Check sheet for the modelled part. Datum: model origin and axes. Units: mm. Face numbers are marked on the shaded views. A direction names the side the tool comes from. Round coordinates to 2 decimals unless told otherwise and drop trailing zeros. Write each loop counter-clockwise with the first axis right and the second up, starting at its lowest first coordinate (ties: lowest second). Pieces come first, ordered by that corner, then holes. Notation, with made-up numbers: (-36, 40) -> (8, 40) arc R26 ccw to (8, 66) -> close; hole circle Ø8 at (69.25, 27). An arc over 180 degrees is marked (long way). Write item = value, one per line.
from build123d import *

# Parameters (mm, degrees)
F2_DEPTH = 3.5
F4_DEPTH = 1
F6_DEPTH = 1.8
F8_DEPTH = 1.2
F9_R     = 3


with BuildPart() as f2:
    # F1 (on Top) → F2 (new body)
    with BuildSketch(Plane.XY):
        Polygon((48.5598316574, 13.5), (5.4801683426, 13.5), (27.0198316574, -13.5), align=None)
    extrude(amount=-F2_DEPTH)

    # F3 (on Top) → F4 (cut)
    with BuildSketch(Plane.XY):
        Polygon((44.7943471372, 11.7882982132), (6.8457046456, 11.7882982132), (25.8198775993, -11.9958558036), align=None)
    extrude(amount=-F4_DEPTH, mode=Mode.SUBTRACT)

    # F5 (on face) → F6 (join)
    with BuildSketch(Plane.XY):
        with BuildLine():
            ThreePointArc((2.8793278964, 3.7278809202), (3.7658696299, 2.8294612951), (4.3820146982, 1.7278809202))
            Line((4.3820146982, 1.7278809202), (14.8715565456, 1.7278809202))
            Line((14.8715565456, 1.7278809202), (17.594606702, -1.6854665007))
            Line((17.594606702, -1.6854665007), (4.3985029231, -1.6854665007))
            ThreePointArc((4.3985029231, -1.6854665007), (3.7999051439, -2.783585132), (2.9334215452, -3.6854665007))
            Line((2.9334215452, -3.6854665007), (19.1901373179, -3.6854665007))
            Line((19.1901373179, -3.6854665007), (25.8198775993, -11.9958558036))
            Line((25.8198775993, -11.9958558036), (44.7943471372, 11.7882982132))
            Line((44.7943471372, 11.7882982132), (6.8457046456, 11.7882982132))
            Line((6.8457046456, 11.7882982132), (13.2760259297, 3.7278809202))
            Line((13.2760259297, 3.7278809202), (2.8793278964, 3.7278809202))
        make_face()
        Polygon((5.4801683426, 13.5), (6.8457046456, 11.7882982132), (44.7943471372, 11.7882982132), (25.8198775993, -11.9958558036), (27.0198316574, -13.5), (48.5598316574, 13.5), align=None)
        with BuildLine():
            Line((-4.3820146982, 1.7278809202), (4.3820146982, 1.7278809202))
            ThreePointArc((4.3820146982, 1.7278809202), (3.7658696299, 2.8294612951), (2.8793278964, 3.7278809202))
            ThreePointArc((2.8793278964, 3.7278809202), (-1.2508065023, 4.5412672663), (-4.3820146982, 1.7278809202))
        make_face()
        with BuildLine():
            ThreePointArc((2.9334215452, -3.6854665007), (3.7999051439, -2.783585132), (4.3985029231, -1.6854665007))
            Line((4.3985029231, -1.6854665007), (-4.3985029231, -1.6854665007))
            ThreePointArc((-4.3985029231, -1.6854665007), (-1.2396031062, -4.5443381728), (2.9334215452, -3.6854665007))
        make_face()
    extrude(amount=F6_DEPTH)

    # F7 (on face) → F8 (join)
    with BuildSketch(Plane.XY.offset(1.8)):
        Polygon((48.5598316574, 13.5), (5.4801683426, 13.5), (13.2760259297, 3.7278809202), (14.8715565456, 1.7278809202), (17.594606702, -1.6854665007), (19.1901373179, -3.6854665007), (27.0198316574, -13.5), align=None)
    extrude(amount=F8_DEPTH)

    # F9
    f9_edges = [f2.edges().sort_by_distance(p)[0] for p in [
        (27.02, 13.5, 3),
        (27.02, 13.5, -3.5),
        (37.789832, 0, 3),
        (37.789832, 0, -3.5),
    ]]
    fillet(f9_edges, radius=F9_R)


solid = f2.part
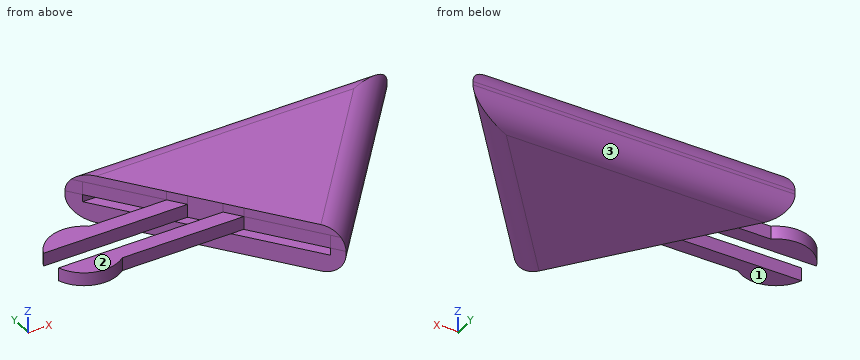
(1) Sectioned sample at B-B on x = 9.5. Enter the section's corners in (y, z), then the cut area to 3 significant figures.
Worked answers:
outline = (-3.69, 0) -> (-1.69, 0) -> (-1.69, 1.8) -> (-3.69, 1.8) -> close; (1.73, 0) -> (3.73, 0) -> (3.73, 1.8) -> (1.73, 1.8) -> close; (8.46, -3.5) -> (10.5, -3.5) arc R3 ccw to (13.5, -0.5) -> (13.5, 0) arc R3 ccw to (10.5, 3) -> (8.46, 3) -> (8.46, 0) -> (11.79, 0) -> (11.79, -1) -> (8.46, -1) -> close
area = 32.8 mm²
(2) Material ranges on L1, parallel to Z at x = 30, y = 0.75; L2, parallel to Y at x = 10, z = 0.5; L3, parallel to Z at x = 16, y = -3.5, recorded low to high. Write a range as [from, to].
Worked answers:
L1 = [-3.5, -1], [0, 3]
L2 = [-3.69, -1.69], [1.73, 3.73], [7.83, 13.46]
L3 = [0, 1.8]
(3) Sectioned sample at D-D on z = 0.5. Enter the section's corners in (x, y), then the cut area to 3 significant figures.
Worked answers:
outline = (-4.4, -1.69) arc R4.71 ccw to (2.93, -3.69) -> (19.19, -3.69) -> (26.99, -13.47) -> (48.47, 13.46) -> (5.51, 13.46) -> (13.28, 3.73) -> (2.88, 3.73) arc R4.71 ccw to (-4.38, 1.73) -> (14.87, 1.73) -> (17.59, -1.69) -> close
area = 666 mm²
(4) Go/stop test with flat-tipped pins: P1, Ø1.4, axis at x = 6, z = 1, coming from the +Y side; P2, Ø12, axis at x = 9, y = -5, coming from the -Z side; P3, Ø2.5, axis at x = 6, y = 4, coming from the +Z side; P4, Ø8, axis at x = 7.5, y = -9.5, coming from the -Z side. Record where each tip stops, or that it passes through.
Worked answers:
P1 = 13.48
P2 = 0
P3 = 1.8
P4 = through
(5) Access from +Z, -Z, +X, -X, +Y, -Y to the whole of each face (thin tool, end or side, straight path). Record for the marked faces 1, 2 and 3.
Worked answers:
face_1 = -X
face_2 = +Z, -X, -Y
face_3 = -Z, +X, -X, +Y
(6) Sectioned sample at C-C on x = 20. Enter the section's corners in (y, z), then the cut area to 3 significant figures.
Worked answers:
outline = (-4.7, -3.5) -> (10.5, -3.5) arc R3 ccw to (13.5, -0.5) -> (13.5, 0) arc R3 ccw to (10.5, 3) -> (-4.7, 3) -> (-4.7, 0) -> (11.79, 0) -> (11.79, -1) -> (-4.7, -1) -> close
area = 98.0 mm²
(7) Sectioned sample at A-A on x = 0. Enter the section's corners in (y, z).
Worked answers:
outline = (-4.71, 0) -> (-1.69, 0) -> (-1.69, 1.8) -> (-4.71, 1.8) -> close; (1.73, 0) -> (4.71, 0) -> (4.71, 1.8) -> (1.73, 1.8) -> close
